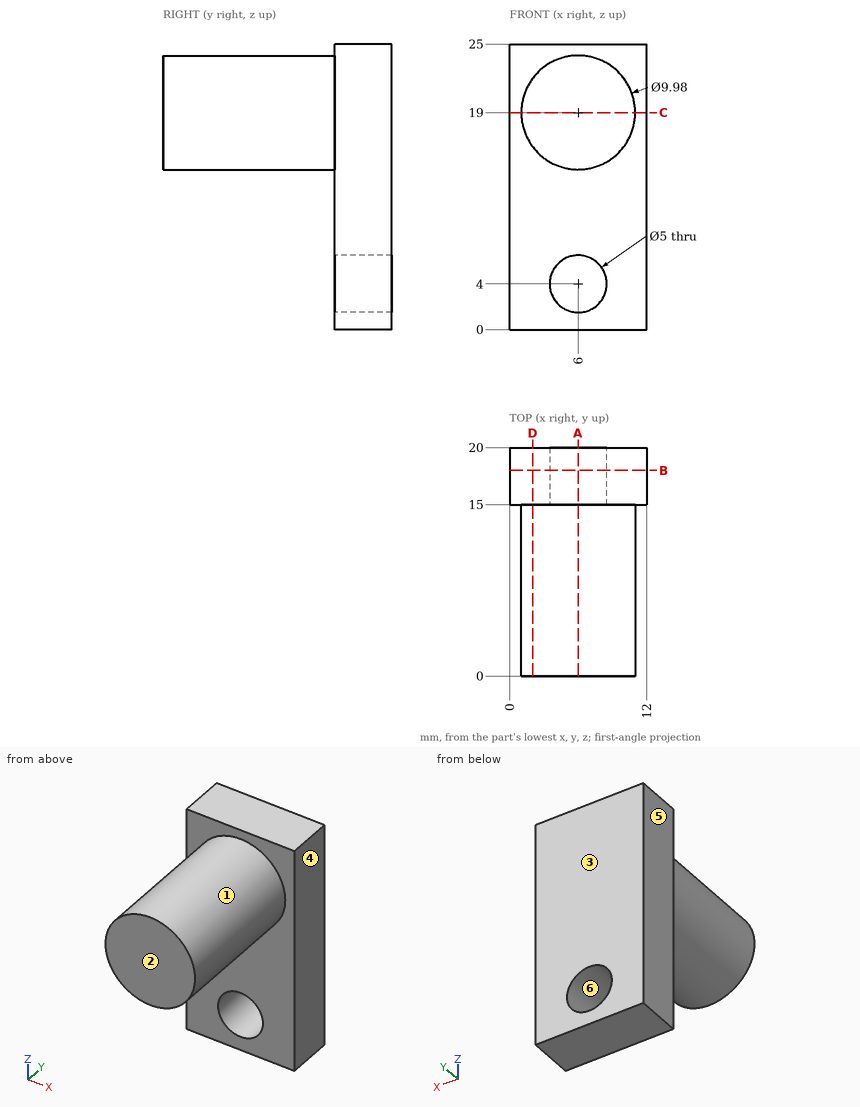
The figure shows three views and two pictorial views of one solid part (mm, origin at its lowest corner). Answer the questions. A direction names the side the tool comes from. Coordinates: 2 decimals unless noted, no trailing zeros. Loops run counter-clockwise (first coordinate to the right, second up) from the corner with the lowest first, then second, coordinate; pieces in that order, holes last. Notation, with made-up numbers: M 18,12.25 L 48,12.25 A16 cw 48,31.25 Z; hole C 5.5,-27 d6. An arc over 180 degrees is marked long. Answer as CSV lines item,"result". Start each with the question number.
(1) The part is cut by section C-C (z = 19). Give the vertices of the cut face in (x, y), and give its area (3 significant figures).
(2) For the marked faces 1 and 2, determine the directions among +Z, -Z, +X, -X, +Y, -Y from which every point of the face is accessible in a straight line to the end or side of a thin tool.
(3) The part is cut by section D-D (x = 2). Give the vertices of the cut face in (y, z).
(4) The part is cut by section A-A (x = 6). Give the vertices of the cut face in (y, z).
(5) The part is cut by section B-B (y = 18). Give the vertices of the cut face in (x, z).
(6) Given pin 1 (6 mm diameter, centred on x = 6, z = 4, fed in from +Y); pin 2 (2 mm diameter, centred on x = 7, y = 7, fed in from +Z); pin 3 (2 mm diameter, centred on x = 10, y = 13.5, fed in from -Z); pin 4 (3.5 mm diameter, centred on x = 4.5, z = 10, fed in from -Y), each flat-ended and moving along its own axis, determine where each tip first touches the part or whether it passes through.
(7) The mould has two halves that part along X. Classify the marked faces 3, 4, 5 and 6: pulls with the +X half, pulls with the -X half, needs draft (parallel to the pull), parting line crosses it, or undercut.
(8) Find the intervals of material crossed by L1, parallel to Y at x = 11.25, z = 16.5; L2, parallel to Z at x = 6, y = 17.6; L3, parallel to Z at x = 8, y = 15.5, in increasing order. Write a range as [from, to].
Determined:
1,outline,"M 0,15 L 1.01,15 L 1.01,0 L 10.99,0 L 10.99,15 L 12,15 L 12,20 L 0,20 Z"
1,area,"210 mm2"
2,face 1,"-Y"
2,face 2,"+Z, -Z, +X, -X, -Y"
3,outline,"M 0,16.02 L 15,16.02 L 15,0 L 20,0 L 20,25 L 15,25 L 15,21.98 L 0,21.98 Z"
4,outline,"M 0,14.01 L 15,14.01 L 15,6.5 L 20,6.5 L 20,25 L 15,25 L 15,23.99 L 0,23.99 Z; M 15,0 L 20,0 L 20,1.5 L 15,1.5 Z"
5,outline,"M 0,0 L 12,0 L 12,25 L 0,25 Z; hole C 6,4 d5"
6,pin 1,"y = 20"
6,pin 2,"z = 23.99"
6,pin 3,"z = 15.01"
6,pin 4,"y = 15"
7,face 3,"needs draft"
7,face 4,"pulls with the +X half"
7,face 5,"pulls with the -X half"
7,face 6,"undercut"
8,L1,"[15, 20]"
8,L2,"[0, 1.5], [6.5, 25]"
8,L3,"[0, 2.5], [5.5, 25]"
